Source: CAD feature listing. Evaluate the final solid. Frame: model axes, mm. A direction names the side the tool comes from. Give positions to 0.01 mm unless a question says otherwise; leave off trailing zeros. Order: outer loops, then holes, each group sorted by start corner. A loop starts at its lowest first (then second) coordinate and runs counter-clockwise, first axis right, second up.
1) Section A-A, the plane x = 13. Return loops of the section in (y, z), plus the area to 3 significant figures.
2) Section B-B, the plane y = 132. Return loops of the section in (x, z).
3) Section C-C, the plane z = 3.1. Return loops of the section in (x, y).
4) Material intervals for line 1 (Y direction, x = 101.5, z = 3.1); line 2 (X direction, y = 142.5, z = 2.05), sorted ascending.
5) Draft query along X for faces 3 (the face through (180, 91, 2)), 4 (the face through (47, 99, 3)), 5 (the face through (0, 91, 2)), 6 (the face through (89, 114, 5)). Return one class per face: released by +X, released by -X, zero draft, split by the parting line, or undercut.
6) Access query for faces 1 (the face through (47, 10, 3)), 2 (the face through (89, 0.04, 2)). Directions: +Z, -Z, +X, -X, +Y, -Y. A direction counts if a zero-diameter tool reaches every point of the face in a straight line with its end or side. Return the directions, or none.
```python
from build123d import *

# Parameters (mm, degrees)
SKETCH_W                     = 180
SKETCH_H                     = 184
PAD_DEPTH                    = 5
SKETCH001_W                  = 75
SKETCH001_H                  = 75
POCKET_DEPTH                 = 5
SKETCH001_LINEARPATTERN_2_W  = 75
SKETCH001_LINEARPATTERN_2_H  = 75
POCKET_LINEARPATTERN_2_DEPTH = 5
LINEARPATTERN001_COUNT       = 2
LINEARPATTERN001_PITCH       = 89


with BuildPart() as part:
    # Sketch → Pad (new body)
    with BuildSketch(Plane.XY):
        with Locations((90, 92.039833)):
            Rectangle(SKETCH_W, SKETCH_H)
    extrude(amount=PAD_DEPTH)

    # Sketch001 (on Face6 of Pad) → Pocket (cut)
    with BuildSketch(Plane.XY.offset(5)):
        with Locations((47.5, 136.5)):
            Rectangle(SKETCH001_W, SKETCH001_H)
    pocket = extrude(amount=-POCKET_DEPTH, mode=Mode.SUBTRACT)

    # Sketch001 LinearPattern 2 → Pocket LinearPattern 2 (cut)
    with BuildSketch(Plane(origin=(85, 0, 5), x_dir=(1, 0, 0), z_dir=(0, 0, 1))):
        with Locations((47.5, 136.5)):
            Rectangle(SKETCH001_LINEARPATTERN_2_W, SKETCH001_LINEARPATTERN_2_H)
    pocket_linearpattern_2 = extrude(amount=-POCKET_LINEARPATTERN_2_DEPTH, mode=Mode.SUBTRACT)

    # LinearPattern001: Pocket, Pocket LinearPattern 2 ×2
    with Locations(*[(0, -i * LINEARPATTERN001_PITCH, 0) for i in range(1, LINEARPATTERN001_COUNT)]):
        add(pocket, mode=Mode.SUBTRACT)
        add(pocket_linearpattern_2, mode=Mode.SUBTRACT)


solid = part.part
```
From the geometry:
1. outline: (0.04, 0) - (10, 0) - (10, 5) - (0.04, 5) - close; (85, 0) - (99, 0) - (99, 5) - (85, 5) - close; (174, 0) - (184.04, 0) - (184.04, 5) - (174, 5) - close
1. area: 170 mm2
2. outline: (0, 0) - (10, 0) - (10, 5) - (0, 5) - close; (85, 0) - (95, 0) - (95, 5) - (85, 5) - close; (170, 0) - (180, 0) - (180, 5) - (170, 5) - close
3. outline: (0, 0.04) - (180, 0.04) - (180, 184.04) - (0, 184.04) - close; hole (10, 10) - (85, 10) - (85, 85) - (10, 85) - close; hole (10, 99) - (85, 99) - (85, 174) - (10, 174) - close; hole (95, 10) - (170, 10) - (170, 85) - (95, 85) - close; hole (95, 99) - (170, 99) - (170, 174) - (95, 174) - close
4. line 1: y = 0.04 to 10, 85 to 99, 174 to 184.04
4. line 2: x = 0 to 10, 85 to 95, 170 to 180
5. face 3: released by +X
5. face 4: undercut
5. face 5: released by -X
5. face 6: zero draft
6. face 1: +Z, -Z
6. face 2: +Z, -Z, +X, -X, -Y
